Read the model definition and answer for the solid it produces. Units are mm, in the model's axes. A direction names the side the tool comes from. Coordinates: 2 decimals unless noted, no trailing zeros. Write each loop counter-clockwise with the first axis right and the second up, starting at its lowest first coordinate (ties: lowest second). Pieces come first, ordered by that corner, then holes. Notation, with made-up numbers: (52, 32) -> (67, 32) arc R7 ccw to (67, 37) -> close; hole circle Ø11 at (82.5, 51). An arc over 180 degrees is marked (long way). Answer in a Markdown table with one row per item. Add a question column.
Item 1: Section A-A on z = -46.5 is taken. Count the separate pieces of the cut face and the enclosed holes in it, then the cut area to 3 significant figures.
Item 2: Section D-D on x = 79 is taken. Write down the section's boundary in (y, z).
Item 3: Section C-C on z = 46.5 is taken. Write down the section's boundary in (x, y).
Item 4: For a pull along Y with two mould halves and no side action, classify faces 6 (the face through (-1, 5, -1)), 7 (the face through (-30.75, -5.12, -36.01)), 8 (the face through (77.017, 2.465, -46.24)) as +Y half, -Y half, draft (parallel to the pull), parting line (faces both ways), or undercut.
Item 5: Given pin 1 Ø4 at (y, z) = (-5.5, -32.5) entering from +X; pin 2 Ø3 at (x, y) = (-61.5, -0.5) entering from -Z; pin 3 Ø6.5 at (y, z) = (-4.5, -44.5) entering from -X; pin 4 Ø5 at (x, y) = (-28.5, -6) entering from +Z, each flat-ended and moving along its own axis, determine where each tip first touches the part or whether it passes through.
Item 6: Which of the six approach directions +Z, -Z, +X, -X, +Y, -Y give full straight-line access (tool end or side, diameter ignored) to faces 1 (the face through (-42.5, -5, -36)), 2 (the face through (42.5, -5, -35)), 3 (the face through (22.5, -5, -35)), 4 (the face through (-32.7, -7.3, -17.5)), 5 (the face through (-1, 0, -1))?
Item 7: Section B-B on y = -5.2 is taken. Write down the section's boundary in (x, z), then the cut area to 3 significant figures.
Item 8: Straight lines are drawn through the part: line 1 (X direction, y = 1.4, z = 46.5); line 2 (X direction, y = -5.2, z = -34.5); line 3 (Y direction, x = -32.5, z = -46). For each, find the intervals that lie inside material, in ascending order. Write a range as from..to.
```python
from build123d import *

# Parameters (mm, degrees)
SKETCH_1_W      = 173
SKETCH_1_H      = 108
SKETCH_1_R      = 2
EXTRUDE_1_DEPTH = 5
SKETCH_2_W      = 20
SKETCH_2_H      = 10.2
SKETCH_2_R      = 1.75
EXTRUDE_2_DEPTH = 30
FILLET_1_R      = 1
EXTRUDE_START   = 6.5
SKETCH_3_R      = 1.75
EXTRUDE_3_DEPTH = 6.5


with BuildPart() as part:
    # 草图1 → 凸台-拉伸1 (new body)
    with BuildSketch(Plane(origin=(0, 0, 0), x_dir=(1, 0, 0), z_dir=(0, 1, 0))):
        Rectangle(SKETCH_1_W, SKETCH_1_H)
        with Locations(Location((-79, 46.5, 0), (0, 0, 270))):
            Circle(SKETCH_1_R, mode=Mode.SUBTRACT)
        with Locations(Location((79, 46.5, 0), (0, 0, 90))):
            Circle(SKETCH_1_R, mode=Mode.SUBTRACT)
        with Locations(Location((79, -46.5, 0), (0, 0, 270))):
            Circle(SKETCH_1_R, mode=Mode.SUBTRACT)
        with Locations(Location((-79, -46.5, 0), (0, 0, 90))):
            Circle(SKETCH_1_R, mode=Mode.SUBTRACT)
    extrude(amount=EXTRUDE_1_DEPTH)

    # 草图2 → 凸台-拉伸2 (add)
    # profile 1 of 2: a face of its own
    with BuildSketch(Plane(origin=(0, 0, -54), x_dir=(-1, 0, 0), z_dir=(0, 0, -1))):
        with Locations((-32.5, -5.1)):
            Rectangle(SKETCH_2_W, SKETCH_2_H)
        with Locations((-32.5, -5.2)):
            Circle(SKETCH_2_R, mode=Mode.SUBTRACT)
    # profile 2 of 2: a face of its own
    with BuildSketch(Plane(origin=(0, 0, -54), x_dir=(-1, 0, 0), z_dir=(0, 0, -1))):
        with Locations((32.5, -5.1)):
            Rectangle(SKETCH_2_W, SKETCH_2_H)
        with Locations((32.5, -5.2)):
            Circle(SKETCH_2_R, mode=Mode.SUBTRACT)
    extrude(amount=-EXTRUDE_2_DEPTH)

    # 圆角1
    fillet_1_edges = [part.edges().sort_by_distance(p)[0] for p in [
        (42.5, -10.2, -39),
        (42.5, 0, -39),
        (22.5, 0, -39),
        (22.5, -10.2, -39),
        (-22.5, -10.2, -39),
        (-22.5, 0, -39),
        (-42.5, 0, -39),
        (-42.5, -10.2, -39),
    ]]
    fillet(fillet_1_edges, radius=FILLET_1_R)

    # 草图3 → 凸台-拉伸3 (add)
    # profile 1 of 2: a face of its own
    with BuildSketch(Plane.XY.offset(-24).offset(EXTRUDE_START)):
        with BuildLine():
            Line((23.5, -10.2), (41.5, -10.2))
            ThreePointArc((41.5, -10.2), (42.207106781, -9.907106781), (42.5, -9.2))
            Line((42.5, -9.2), (42.5, -1))
            ThreePointArc((42.5, -1), (42.792893219, -0.292893219), (43.5, 0))
            Line((43.5, 0), (21.5, 0))
            ThreePointArc((21.5, 0), (22.207106781, -0.292893219), (22.5, -1))
            Line((22.5, -1), (22.5, -9.2))
            ThreePointArc((22.5, -9.2), (22.792893219, -9.907106781), (23.5, -10.2))
        make_face()
        with Locations(Location((32.5, -5.2, 0), (0, 0, 180))):
            Circle(SKETCH_3_R, mode=Mode.SUBTRACT)
    # profile 2 of 2: a face of its own
    with BuildSketch(Plane.XY.offset(-24).offset(EXTRUDE_START)):
        with BuildLine():
            Line((-41.5, -10.2), (-23.5, -10.2))
            ThreePointArc((-23.5, -10.2), (-22.792893219, -9.907106781), (-22.5, -9.2))
            Line((-22.5, -9.2), (-22.5, -1))
            ThreePointArc((-22.5, -1), (-22.207106781, -0.292893219), (-21.5, 0))
            Line((-21.5, 0), (-43.5, 0))
            ThreePointArc((-43.5, 0), (-42.792893219, -0.292893219), (-42.5, -1))
            Line((-42.5, -1), (-42.5, -9.2))
            ThreePointArc((-42.5, -9.2), (-42.207106781, -9.907106781), (-41.5, -10.2))
        make_face()
        with Locations(Location((-32.5, -5.2, 0), (0, 0, 180))):
            Circle(SKETCH_3_R, mode=Mode.SUBTRACT)
    extrude(amount=-EXTRUDE_3_DEPTH)


solid = part.part
```
Results below:
| question | item | result |
|---|---|---|
| 1 | separate pieces | 3 |
| 1 | enclosed holes | 2 |
| 1 | area | 1,210 mm2 |
| 2 | outline | (0, -54) -> (5, -54) -> (5, -48.5) -> (0, -48.5) -> close; (0, -44.5) -> (5, -44.5) -> (5, 44.5) -> (0, 44.5) -> close; (0, 48.5) -> (5, 48.5) -> (5, 54) -> (0, 54) -> close |
| 3 | outline | (-86.5, 0) -> (-81, 0) -> (-81, 5) -> (-86.5, 5) -> close; (-77, 0) -> (77, 0) -> (77, 5) -> (-77, 5) -> close; (81, 0) -> (86.5, 0) -> (86.5, 5) -> (81, 5) -> close |
| 4 | face 6 | +Y half |
| 4 | face 7 | undercut |
| 4 | face 8 | draft |
| 5 | pin 1 | stops at x = 42.5 |
| 5 | pin 2 | stops at z = -54 |
| 5 | pin 3 | stops at x = -42.5 |
| 5 | pin 4 | stops at z = -17.5 |
| 6 | face 1 | +Z, -Z, -X, -Y |
| 6 | face 2 | +Z, -Z, +X, -Y |
| 6 | face 3 | +Z, -Z, -Y |
| 6 | face 4 | +Z, +X, -X, -Y |
| 6 | face 5 | +Z, -Y |
| 7 | outline | (-42.5, -54) -> (-34.25, -54) -> (-34.25, -17.5) -> (-42.5, -17.5) -> close; (-30.75, -54) -> (-22.5, -54) -> (-22.5, -17.5) -> (-30.75, -17.5) -> close; (22.5, -54) -> (30.75, -54) -> (30.75, -17.5) -> (22.5, -17.5) -> close; (34.25, -54) -> (42.5, -54) -> (42.5, -17.5) -> (34.25, -17.5) -> close |
| 7 | area | 1,200 mm2 |
| 8 | line 1 | x = -86.5..-81, -77..77, 81..86.5 |
| 8 | line 2 | x = -42.5..-34.25, -30.75..-22.5, 22.5..30.75, 34.25..42.5 |
| 8 | line 3 | y = -10.2..-6.95, -3.45..5 |
